```python
from build123d import *

# Parameters (mm, degrees)
SKETCH_1_W                   = 20
SKETCH_1_H                   = 23
EXTRUDE_1_DEPTH              = 12.5
CUT_EXTRUDE_1_DEPTH          = 26.5
SKETCH_3_W                   = 20
SKETCH_3_H                   = 10
CUT_EXTRUDE_2_DEPTH          = 8.5
HOLE_WIZARD_M3_1_D           = 3.2
HOLE_WIZARD_M3_1_CBORE_D     = 5.2
HOLE_WIZARD_M3_1_CBORE_DEPTH = 1.5


with BuildPart() as part:
    # 草图1 → 凸台-拉伸1 (new body)
    with BuildSketch(Plane.XY):
        with Locations((120, 93.5)):
            Rectangle(SKETCH_1_W, SKETCH_1_H)
    extrude(amount=EXTRUDE_1_DEPTH)

    # 草图2 → 切除-拉伸1 (cut)
    with BuildSketch(Plane(origin=(0, 105, 0), x_dir=(1, 0, 0), z_dir=(0, 1, 0))):
        with BuildLine():
            Line((129.40254033, -8.557993857), (130, -6.161714003))
            Line((130, -6.161714003), (130, -12.5))
            Line((130, -12.5), (124.357002553, -12.5))
            ThreePointArc((124.357002553, -12.5), (127.558442225, -11.397655919), (129.40254033, -8.557993857))
        make_face()
    extrude(amount=-CUT_EXTRUDE_1_DEPTH, mode=Mode.SUBTRACT)

    # 草图3 → 切除-拉伸2 (cut)
    with BuildSketch(Plane.XY.offset(12.5)):
        with Locations((120, 93.5)):
            Rectangle(SKETCH_3_W, SKETCH_3_H)
    extrude(amount=-CUT_EXTRUDE_2_DEPTH, mode=Mode.SUBTRACT)

    # M3 六角头螺栓的柱形沉头孔1 (through all)
    with Locations(Plane.XY.offset(4)):
        with Locations((115, 93.5), (123, 93.5)):
            CounterBoreHole(HOLE_WIZARD_M3_1_D / 2, HOLE_WIZARD_M3_1_CBORE_D / 2, HOLE_WIZARD_M3_1_CBORE_DEPTH)


solid = part.part
```
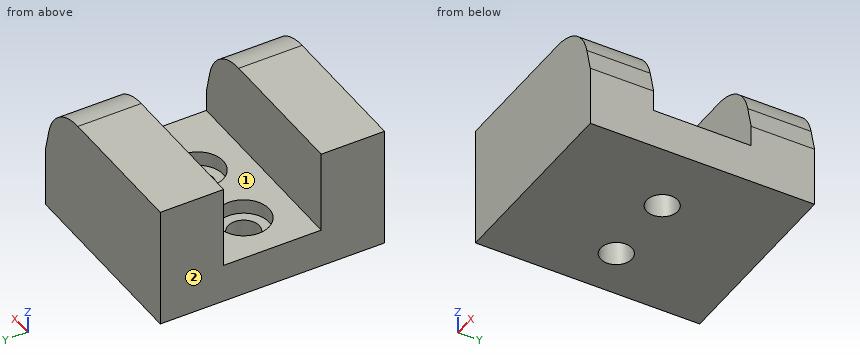
Input: part model. Units: mm. Frame: model coordinates. Face numbers are marked on the shaded views. A direction names the side the tool comes from. Round coordinates to 2 decimals unless told otherwise and drop trailing zeros. Loops run counter-clockwise (first coordinate to the right, second up) from the corner with the lowest first, then second, coordinate; pieces in that order, holes last. Notation, with made-up numbers: (60.25, 68) -> (87.25, 68) arc R31 cw to (87.25, 105) -> close; hole circle Ø6 at (-8.5, 35). An arc over 180 degrees is marked (long way). Use one line per item in the form item = value. Start each with the question number.
Item 1: Section query D-D on y = 83.5. Return the cut outline in (x, z), then the cut area to 3 significant figures.
Item 2: Section query C-C on x = 115. Return the cut outline in (y, z), then the cut area to 3 significant figures.
Item 3: Section query B-B on z = 6.75. Return the cut outline in (x, y).
Item 4: Contact query for flat-ended pins moving along their axis: pin 1 Ø7 at (x, y) = (123, 93.5) entering from -Z; pin 2 Ø4 at (x, y) = (115, 93.5) entering from +Z; pin 3 Ø3 at (x, y) = (117, 91.5) entering from +Z. Output: stop coordinate, or through.
Item 5: Section query A-A on y = 93.5. Return the cut outline in (x, z).
Item 6: Material intervals for L1, parallel to X at y = 93.5, z = 0.95; L2, parallel to Y at x = 118, z = 7; L3, parallel to Y at x = 123, z = 3.4, sorted ascending. Write a range as from..to.
Item 7: Set-up query: the marked faces 1 and 2. Return all of +Z, -Z, +X, -X, +Y, -Y with unobstructed straight access to the full face (end or side cutting, diameter ignored); none if empty.
Ans:
q1.outline = (110, 0) -> (130, 0) -> (130, 6.16) -> (129.4, 8.56) arc R5.2 ccw to (124.36, 12.5) -> (110, 12.5) -> close
q1.area = 242 mm^2
q2.outline = (82, 0) -> (91.9, 0) -> (91.9, 2.5) -> (90.9, 2.5) -> (90.9, 4) -> (88.5, 4) -> (88.5, 12.5) -> (82, 12.5) -> close; (95.1, 0) -> (105, 0) -> (105, 12.5) -> (98.5, 12.5) -> (98.5, 4) -> (96.1, 4) -> (96.1, 2.5) -> (95.1, 2.5) -> close
q2.area = 187 mm^2
q3.outline = (110, 82) -> (129.85, 82) -> (129.85, 88.5) -> (110, 88.5) -> close; (110, 98.5) -> (129.85, 98.5) -> (129.85, 105) -> (110, 105) -> close
q4.pin_1 = 0
q4.pin_2 = 2.5
q4.pin_3 = 4
q5.outline = (110, 0) -> (113.4, 0) -> (113.4, 2.5) -> (112.4, 2.5) -> (112.4, 4) -> (110, 4) -> close; (116.6, 0) -> (121.4, 0) -> (121.4, 2.5) -> (120.4, 2.5) -> (120.4, 4) -> (117.6, 4) -> (117.6, 2.5) -> (116.6, 2.5) -> close; (124.6, 0) -> (130, 0) -> (130, 4) -> (125.6, 4) -> (125.6, 2.5) -> (124.6, 2.5) -> close
q6.L1 = 110..113.4, 116.6..121.4, 124.6..130
q6.L2 = 82..88.5, 98.5..105
q6.L3 = 82..90.9, 96.1..105
q7.face_1 = +Z, +X, -X
q7.face_2 = +Z, -Z, -X, +Y, -Y
